Could you check a few things on this model? Use its own coordinates, in mm. A direction names the side the tool comes from. Give positions to 0.01 mm unless a question says otherwise; leave off trailing zeros. Order: outer loops, then holes, each group sorted by start corner. A loop starts at its lowest first (then second) coordinate and runs counter-clockwise, first axis right, second up. Notation, with made-up numbers: (50.5, 85) -> (68.5, 85) arc R28 cw to (68.5, 122) -> close; hole circle Ø2 at (-1.75, -24). An arc over 180 degrees is marked (long way). One line per item, written item: value.
Autodesk Fusion 360 part; units mm, degrees
sketch "Sketch1" plane through (0, 0, 0) normal (0, 1, 0) x (1, 0, 0)
  circle A0 centre (0, 0) radius 2.5
  circle A1 centre (0, 0) radius 3.5
  dimension "d1" = 5
  dimension "d2" = 7
extrude "Extrude2" add sketch "Sketch1" along normal blind 1

Autodesk Fusion 360 part; units mm, degrees
sketch "Sketch1" plane through (0, 0, 0) normal (0, 1, 0) x (1, 0, 0)
  circle A0 centre (0, 0) radius 2.5
  circle A1 centre (0, 0) radius 6.125
  circle A2 centre (0, 0) radius 7.5
  dimension "d1" = 5
  dimension "d2" = 12.25
  dimension "d3" = 15
extrude "Extrude1" add sketch "Sketch1" along normal blind 10 contours A1
extrude "Extrude2" add sketch "Sketch1" along normal blind 1.5 contours A2
extrude "Extrude3" add sketch "Sketch1" against normal blind 1.5 from surface at 10 contours A2
1) For faces 5 (the flat face through (-3, 1.5, 6)), 6 (the cylindrical face through (-7.493, 9.26, -0.33)), which set-ups out of +Z, -Z, +X, -X, +Y, -Y let a thin tool reach every point of the face, with its end or its side?
Answer below:
face 5: none
face 6: +Y, -Y
2) Suppose I cut it at D-D, the plane y = 3.75. Write out the boundary of the cut face in (x, z) (3 decimals).
Answer below:
outline: circle Ø12.25 at (0, 0); hole circle Ø5 at (0, 0)
3) Suppose I cut it at C-C, the plane z = 4.25. Write out the boundary of the cut face in (x, y), then the cut area to 3 significant figures.
Answer below:
outline: (-6.18, 0) -> (6.18, 0) -> (6.18, 1.5) -> (4.41, 1.5) -> (4.41, 8.5) -> (6.18, 8.5) -> (6.18, 10) -> (-6.18, 10) -> (-6.18, 8.5) -> (-4.41, 8.5) -> (-4.41, 1.5) -> (-6.18, 1.5) -> close
area: 98.8 mm2
4) Suppose I cut it at B-B, the plane x = 0. Write out the boundary of the cut face in (y, z) (3 decimals).
Answer below:
outline: (0, -7.5) -> (1.5, -7.5) -> (1.5, -6.125) -> (8.5, -6.125) -> (8.5, -7.5) -> (10, -7.5) -> (10, -2.5) -> (1, -2.5) -> (1, 2.5) -> (10, 2.5) -> (10, 7.5) -> (8.5, 7.5) -> (8.5, 6.125) -> (1.5, 6.125) -> (1.5, 7.5) -> (0, 7.5) -> close
5) For P1, Ø1.5, axis at x = 1, z = -1, coming from the +Y side; P2, Ø1, axis at y = 4.5, z = 2, coming from the +X side; P3, Ø1.5, axis at x = 2, y = 3, coming from the -Z side, each with a flat end and sliding along its axis, tell me the tip position at first contact or that it passes through.
Answer below:
P1: stops at y = 1
P2: stops at x = 5.94
P3: stops at z = -6
6) If I drill on line 1 along X through (y, z) = (4, 0) (3 decimals); line 2 along Y through (x, z) = (-6.25, 2.5), over which ranges is the centre line in solid material (lowest first)?
Answer below:
line 1: x = -6.125 to -2.5, 2.5 to 6.125
line 2: y = 0 to 1.5, 8.5 to 10
7) We'd pull the mould along X, two halves only. Please class faces 1 (the flat face through (0, 1, 0)), 2 (the cylindrical face through (-7.493, 0.74, 0.33)), 3 (the flat face through (-3, 8.5, 6)), 4 (the cylindrical face through (-0.54, 5.44, -2.44)): +X half, -X half, draft (parallel to the pull), parting line (faces both ways), or undercut.
Answer below:
face 1: undercut
face 2: parting line
face 3: draft
face 4: undercut
8) Suppose I cut it at A-A, the plane z = 6.75. Write out the boundary of the cut face in (x, y).
Answer below:
outline: (-3.27, 0) -> (3.27, 0) -> (3.27, 1.5) -> (-3.27, 1.5) -> close; (-3.27, 8.5) -> (3.27, 8.5) -> (3.27, 10) -> (-3.27, 10) -> close
